Could you check a few things on this model? Use its own coordinates, in mm. A direction names the side the tool comes from. Give positions to 0.01 mm unless a question says otherwise; leave off trailing zeros. Write each loop counter-clockwise with the first axis right and the second up, starting at its lowest first coordinate (ties: lowest second). Pieces come first, ordered by that corner, then holes. Notation, with made-up numbers: M -3,44.25 L 21,44.25 A21 cw 21,76.25 Z; hole C 1,41.25 d10. An arc over 180 degrees is marked long. One line per item, written item: value.
Autodesk Fusion 360 part; units mm, degrees
sketch "Sketch1" plane through (0, 0, 0) normal (0, 1, 0) x (1, 0, 0)
  circle A0 centre (0, 0) radius 15
  circle A1 centre (0, 0) radius 25
  line L0 (0, 0) -> (0, -54.75) construction
  circle A2 centre (0, -54.75) radius 2.435
  line L1 (4.5611, -54.75) -> (2.2805, -50.8)
  line L2 (2.2805, -50.8) -> (-2.2805, -50.8)
  line L3 (-2.2805, -50.8) -> (-4.5611, -54.75)
  line L4 (-4.5611, -54.75) -> (-2.2805, -58.7)
  line L5 (-2.2805, -58.7) -> (2.2805, -58.7)
  line L6 (2.2805, -58.7) -> (4.5611, -54.75)
  line L7 (-10, -22.9129) -> (-10, -54.75)
  arc A3 (-10, -54.75) -> (10, -54.75) centre (0, -54.75) ccw
  line L8 (10, -54.75) -> (10, -22.9129)
  line L9 (0, 0) -> (47.4149, 27.375) construction
  line L10 (45.1344, 31.325) -> (42.8538, 27.375)
  circle A4 centre (47.4149, 27.375) radius 2.435
  line L11 (51.976, 27.375) -> (49.6954, 31.325)
  line L12 (42.8538, 27.375) -> (45.1344, 23.425)
  line L13 (49.6954, 23.425) -> (51.976, 27.375)
  line L14 (45.1344, 23.425) -> (49.6954, 23.425)
  arc A5 (52.4149, 18.7147) -> (42.4149, 36.0353) centre (47.4149, 27.375) ccw
  line L15 (49.6954, 31.325) -> (45.1344, 31.325)
  line L16 (42.4149, 36.0353) -> (14.8431, 20.1167)
  line L17 (24.8431, 2.7962) -> (52.4149, 18.7147)
  line L18 (0, 0) -> (-47.4149, 27.375) construction
  line L19 (-49.6954, 23.425) -> (-45.1344, 23.425)
  circle A6 centre (-47.4149, 27.375) radius 2.435
  line L20 (-49.6954, 31.325) -> (-51.976, 27.375)
  line L21 (-45.1344, 23.425) -> (-42.8538, 27.375)
  line L22 (-45.1344, 31.325) -> (-49.6954, 31.325)
  line L23 (-42.8538, 27.375) -> (-45.1344, 31.325)
  arc A7 (-42.4149, 36.0353) -> (-52.4149, 18.7147) centre (-47.4149, 27.375) ccw
  line L24 (-51.976, 27.375) -> (-49.6954, 23.425)
  line L25 (-52.4149, 18.7147) -> (-24.8431, 2.7962)
  line L26 (-14.8431, 20.1167) -> (-42.4149, 36.0353)
  point P0 (0, -54.75)
  point P1 (47.4149, 27.375)
  point P2 (-47.4149, 27.375)
  dimension "d1" = 30
  dimension "d2" = 50
  dimension "d3" = 7.9
  dimension "d4" = 4.87
  dimension "d5" = 50.8
  dimension "d6" = 10
  dimension "d8" = 360
extrude "Extrude1" add sketch "Sketch1" along normal blind 4 contours A1 | A1 A5 L16 L17 | A1 L7 A3 L8 | A1 A7 L25 L26 | L1 L2 L3 L4 L5 L6 | L10 L11 L12 L13 L14 L15 | L19 L20 L21 L22 L23 L24
sketch "Sketch2" plane through (0, 0, 0) normal (0, -1, 0) x (1, 0, 0)
  circle A0 centre (0, 0) radius 15
  circle A1 centre (47.4149, -27.375) radius 2.435
  circle A2 centre (0, 54.75) radius 2.435
  circle A3 centre (-47.4149, -27.375) radius 2.435
  line L0 (-42.4149, -36.0353) -> (-14.8431, -20.1167)
  arc A4 (-14.8431, -20.1167) -> (14.8431, -20.1167) centre (0, 0) ccw
  line L1 (14.8431, -20.1167) -> (42.4149, -36.0353)
  arc A5 (42.4149, -36.0353) -> (52.4149, -18.7147) centre (47.4149, -27.375) ccw
  line L2 (52.4149, -18.7147) -> (24.8431, -2.7962)
  arc A6 (24.8431, -2.7962) -> (10, 22.9129) centre (0, 0) ccw
  line L3 (10, 22.9129) -> (10, 54.75)
  arc A7 (10, 54.75) -> (-10, 54.75) centre (0, 54.75) ccw
  line L4 (-10, 54.75) -> (-10, 22.9129)
  arc A8 (-10, 22.9129) -> (-24.8431, -2.7962) centre (0, 0) ccw
  line L5 (-24.8431, -2.7962) -> (-52.4149, -18.7147)
  arc A9 (-52.4149, -18.7147) -> (-42.4149, -36.0353) centre (-47.4149, -27.375) ccw
  line L6 (2.2372, 50.875) -> (4.4745, 54.75)
  line L7 (4.4745, 54.75) -> (2.2372, 58.625)
  line L8 (2.2372, 58.625) -> (-2.2372, 58.625)
  line L9 (-2.2372, 58.625) -> (-4.4745, 54.75)
  line L10 (-4.4745, 54.75) -> (-2.2372, 50.875)
  line L11 (-2.2372, 50.875) -> (2.2372, 50.875)
  line L12 (-51.8894, -27.375) -> (-49.6521, -31.25)
  line L13 (-45.1777, -23.5) -> (-49.6521, -23.5)
  line L14 (-42.9404, -27.375) -> (-45.1777, -23.5)
  line L15 (-49.6521, -31.25) -> (-45.1777, -31.25)
  circle A10 centre (-47.4149, -27.375) radius 2.435
  line L16 (-45.1777, -31.25) -> (-42.9404, -27.375)
  line L17 (-49.6521, -23.5) -> (-51.8894, -27.375)
  line L18 (49.6521, -31.25) -> (51.8894, -27.375)
  line L19 (42.9404, -27.375) -> (45.1777, -31.25)
  line L20 (45.1777, -23.5) -> (42.9404, -27.375)
  line L21 (51.8894, -27.375) -> (49.6521, -23.5)
  circle A11 centre (47.4149, -27.375) radius 2.435
  line L22 (49.6521, -23.5) -> (45.1777, -23.5)
  line L23 (45.1777, -31.25) -> (49.6521, -31.25)
  point P0 (0, 54.75)
  point P1 (-47.4149, -27.375)
  point P2 (47.4149, -27.375)
  dimension "d11" = 7.75
  dimension "d13" = 360
extrude "Extrude2" add sketch "Sketch2" along normal blind 9 contours L6 L7 L8 L9 L10 L11 | L12 L13 L14 L15 L16 L17 | L18 L19 L20 L21 L22 L23
sketch "Sketch3" plane through (0, 4, 0) normal (0, 1, 0) x (-1, 0, 0)
  circle A0 centre (0, 0) radius 15
  circle A1 centre (-47.4149, -27.375) radius 2.435
  circle A2 centre (0, 54.75) radius 2.435
  circle A3 centre (47.4149, -27.375) radius 2.435
  line L0 (14.8431, -20.1167) -> (42.4149, -36.0353)
  arc A4 (42.4149, -36.0353) -> (52.4149, -18.7147) centre (47.4149, -27.375) ccw
  line L1 (52.4149, -18.7147) -> (24.8431, -2.7962)
  arc A5 (24.8431, -2.7962) -> (10, 22.9129) centre (0, 0) ccw
  line L2 (10, 22.9129) -> (10, 54.75)
  arc A6 (10, 54.75) -> (-10, 54.75) centre (0, 54.75) ccw
  line L3 (-10, 54.75) -> (-10, 22.9129)
  arc A7 (-10, 22.9129) -> (-24.8431, -2.7962) centre (0, 0) ccw
  line L4 (-24.8431, -2.7962) -> (-52.4149, -18.7147)
  arc A8 (-52.4149, -18.7147) -> (-42.4149, -36.0353) centre (-47.4149, -27.375) ccw
  line L5 (-42.4149, -36.0353) -> (-14.8431, -20.1167)
  arc A9 (-14.8431, -20.1167) -> (14.8431, -20.1167) centre (0, 0) ccw
  line L6 (0, 54.75) -> (0, 15) construction
  circle A10 centre (0, 23) radius 3
  circle A11 centre (0, 23) radius 1.575
  circle A12 centre (-19.9186, -11.5) radius 3
  circle A13 centre (-19.9186, -11.5) radius 1.575
  circle A14 centre (19.9186, -11.5) radius 3
  circle A15 centre (19.9186, -11.5) radius 1.575
  dimension "d16" = 8
  dimension "d17" = 6
  dimension "d18" = 3.15
  dimension "d20" = 360
extrude "Extrude3" add sketch "Sketch3" along normal blind 8 contours A10 | A12 | A14
extrude "Extrude4" cut 3 faces at (0.5191, 4, 23.8992) (-20.3985, 4, -11.9453) (20.3916, 4, -11.4183) along direction (0, 1, 0) up to surface end surface through (0, 0, 0) normal (0, -1, 0) offset 0
sketch "Sketch4" plane through (0, 0, 0) normal (0, -1, 0) x (1, 0, 0)
  circle A0 centre (-19.9186, -11.5) radius 1.575
  circle A1 centre (0, 23) radius 1.575
  circle A2 centre (19.9186, -11.5) radius 1.575
  line L0 (-2.2372, 50.875) -> (-4.4745, 54.75)
  line L1 (-4.4745, 54.75) -> (-2.2372, 58.625)
  line L2 (-2.2372, 58.625) -> (2.2372, 58.625)
  line L3 (2.2372, 58.625) -> (4.4745, 54.75)
  line L4 (4.4745, 54.75) -> (2.2372, 50.875)
  line L5 (2.2372, 50.875) -> (-2.2372, 50.875)
  line L6 (-49.6521, -23.5) -> (-45.1777, -23.5)
  line L7 (-45.1777, -23.5) -> (-42.9404, -27.375)
  line L8 (-42.9404, -27.375) -> (-45.1777, -31.25)
  line L9 (-45.1777, -31.25) -> (-49.6521, -31.25)
  line L10 (-49.6521, -31.25) -> (-51.8894, -27.375)
  line L11 (-51.8894, -27.375) -> (-49.6521, -23.5)
  line L12 (45.1777, -31.25) -> (42.9404, -27.375)
  line L13 (42.9404, -27.375) -> (45.1777, -23.5)
  line L14 (45.1777, -23.5) -> (49.6521, -23.5)
  line L15 (49.6521, -23.5) -> (51.8894, -27.375)
  line L16 (51.8894, -27.375) -> (49.6521, -31.25)
  line L17 (49.6521, -31.25) -> (45.1777, -31.25)
  circle A3 centre (0, 0) radius 15
  line L18 (-42.4149, -36.0353) -> (-14.8431, -20.1167)
  arc A4 (-14.8431, -20.1167) -> (14.8431, -20.1167) centre (0, 0) ccw
  line L19 (14.8431, -20.1167) -> (42.4149, -36.0353)
  arc A5 (42.4149, -36.0353) -> (52.4149, -18.7147) centre (47.4149, -27.375) ccw
  line L20 (52.4149, -18.7147) -> (24.8431, -2.7962)
  arc A6 (24.8431, -2.7962) -> (10, 22.9129) centre (0, 0) ccw
  line L21 (10, 22.9129) -> (10, 54.75)
  arc A7 (10, 54.75) -> (-10, 54.75) centre (0, 54.75) ccw
  line L22 (-10, 54.75) -> (-10, 22.9129)
  arc A8 (-10, 22.9129) -> (-24.8431, -2.7962) centre (0, 0) ccw
  line L23 (-24.8431, -2.7962) -> (-52.4149, -18.7147)
  arc A9 (-52.4149, -18.7147) -> (-42.4149, -36.0353) centre (-47.4149, -27.375) ccw
  line L24 (18.2876, -14.325) -> (21.5496, -14.325)
  line L25 (21.5496, -14.325) -> (23.1806, -11.5)
  line L26 (23.1806, -11.5) -> (21.5496, -8.675)
  line L27 (21.5496, -8.675) -> (18.2876, -8.675)
  line L28 (18.2876, -8.675) -> (16.6566, -11.5)
  line L29 (16.6566, -11.5) -> (18.2876, -14.325)
  line L30 (3.262, 23) -> (1.631, 25.825)
  line L31 (1.631, 20.175) -> (3.262, 23)
  line L32 (1.631, 25.825) -> (-1.631, 25.825)
  line L33 (-1.631, 25.825) -> (-3.262, 23)
  line L34 (-3.262, 23) -> (-1.631, 20.175)
  line L35 (-1.631, 20.175) -> (1.631, 20.175)
  line L36 (-21.5496, -8.675) -> (-23.1806, -11.5)
  line L37 (-18.2876, -8.675) -> (-21.5496, -8.675)
  line L38 (-23.1806, -11.5) -> (-21.5496, -14.325)
  line L39 (-21.5496, -14.325) -> (-18.2876, -14.325)
  line L40 (-18.2876, -14.325) -> (-16.6566, -11.5)
  line L41 (-16.6566, -11.5) -> (-18.2876, -8.675)
  point P0 (19.9186, -11.5)
  point P1 (0, 23)
  point P2 (-19.9186, -11.5)
  dimension "d25" = 5.65
  dimension "d27" = 360
extrude "Extrude5" cut sketch "Sketch4" against normal up to surface (3 mm away) contours L24 L25 L26 L27 L28 L29 | L30 L31 L32 L33 L34 L35 | L36 L37 L38 L39 L40 L41
1) We'd pull the mould along Z, two halves only. Please class faces 6 (the face through (17.46, 1.48, -12.89)), 7 (the face through (-20, 1, -14.325)), 8 (the face through (-44.043, -4.437, -25.465)), 9 (the face through (3.34, -4.437, 52.785)): pulls with the +Z half, pulls with the -Z half, needs draft (parallel to the pull), parting line crosses it, or undercut.
Outcome:
face 6: undercut
face 7: undercut
face 8: pulls with the +Z half
face 9: pulls with the -Z half
2) If we section it at B-B, the plane z = 0: Write out the boundary of the cut face in (x, y), then the cut area to 3 significant figures.
Outcome:
outline: M -25,0 L -15,0 L -15,4 L -25,4 Z; M 15,0 L 25,0 L 25,4 L 15,4 Z
area: 80.0 mm^2
3) If we section it at C-C, the plane x = -7: Write out the boundary of the cut face in (y, z), then the cut area to 3 significant figures.
Outcome:
outline: M 0,-24 L 4,-24 L 4,-13.27 L 0,-13.27 Z; M 0,13.27 L 4,13.27 L 4,61.89 L 0,61.89 Z
area: 237 mm^2
4) If we section it at D-D, the plane y = -4: Give the number of separate pieces and of enclosed holes in the cut face, then the cut area to 3 significant figures.
Outcome:
separate pieces: 3
enclosed holes: 3
area: 100 mm^2
5) If we section it at A-A, the plane y = 8.75: Write out the boundary of the cut face in (x, z) (3 decimals), then the cut area to 3 significant figures.
Outcome:
outline: C -19.919,-11.5 d6; C 0,23 d6; C 19.919,-11.5 d6; hole C -19.919,-11.5 d3.15; hole C 0,23 d3.15; hole C 19.919,-11.5 d3.15
area: 61.4 mm^2
6) On a 3-axis mill with a long thin cutter (end or side, diameter ignored), from which of +Z, -Z, +X, -X, +Y, -Y can I reach the whole of each face in a straight line? I mean faces 1 (the face through (44.982, -2.591, -27.268)), 2 (the face through (-1.3, 12, 21.7)), 3 (the face through (28.822, 1.972, -28.187)), 4 (the face through (50.755, -4.437, -29.34)), 5 (the face through (-20, 1, -8.675)). Say none if no direction works.
Outcome:
face 1: +Y, -Y
face 2: +Z, -Z, +X, -X, +Y
face 3: -Z, +Y, -Y
face 4: -Z, +X, -Y
face 5: -Y
7) I'm going to push flat-ended pins straight in: pin 1 (1 mm diameter, centred on x = 14.5, y = 5.5, fed in from -Z); pin 2 (2 mm diameter, centred on x = -48, y = -4, fed in from -Z); pin 3 (3 mm diameter, centred on y = 1, z = 41.5, fed in from +X); pin 4 (8 mm diameter, centred on x = -5.5, y = 8.5, fed in from +Z). Where does each tip first touch, or does it pass through?
Outcome:
pin 1: passes through
pin 2: stops at z = -31.25
pin 3: stops at x = 10
pin 4: stops at z = 25.6
8) Please list where these lines run through material, in increasing order: L1, parallel to X at y = 2.15, z = 0; L2, parallel to X at y = -0.5, z = 54.75 (1 decimal); L3, parallel to X at y = 3, z = 39.5. Write a range as from..to.
Outcome:
L1: x = -25..-15, 15..25
L2: x = -4.5..-2.4, 2.4..4.5
L3: x = -10..10
